```python
from build123d import *

# Parameters (mm, degrees)
SKETCH1_W           = 40
SKETCH1_H           = 40
BOSS_EXTRUDE1_DEPTH = 30
SKETCH2_R           = 19
CUT_EXTRUDE1_DEPTH  = 30
CUT_EXTRUDE1_TAPER  = 6
SKETCH3_R           = 1.5
CUT_EXTRUDE2_DEPTH  = 15
SKETCH4_W           = 24
SKETCH4_H           = 15
CUT_EXTRUDE3_DEPTH  = 41
SKETCH5_W           = 30
SKETCH5_H           = 25
CUT_EXTRUDE4_DEPTH  = 15
SKETCH7_R           = 1.75
BOSS_EXTRUDE2_DEPTH = 5
FILLET1_R           = 10
FILLET2_R           = 10


with BuildPart() as part:
    # Sketch1 → Boss-Extrude1 (new body)
    with BuildSketch(Plane(origin=(0, 0, 0), x_dir=(1, 0, 0), z_dir=(0, 1, 0))):
        Rectangle(SKETCH1_W, SKETCH1_H)
    extrude(amount=BOSS_EXTRUDE1_DEPTH)

    # Sketch2 → Cut-Extrude1 (cut)
    with BuildSketch(Plane(origin=(0, 30, 0), x_dir=(1, 0, 0), z_dir=(0, 1, 0))):
        Circle(SKETCH2_R)
    extrude(amount=-CUT_EXTRUDE1_DEPTH, taper=CUT_EXTRUDE1_TAPER, mode=Mode.SUBTRACT)

    # Sketch3 → Cut-Extrude2 (cut)
    with BuildSketch(Plane(origin=(0, 30, 0), x_dir=(1, 0, 0), z_dir=(0, 1, 0))):
        with Locations((-15.810907627, 15.810907627)):
            Circle(SKETCH3_R)
        with Locations((16.189092373, 15.810907627)):
            Circle(SKETCH3_R)
        with Locations((16.189092373, -16.189092373)):
            Circle(SKETCH3_R)
        with Locations((-15.810907627, -16.189092373)):
            Circle(SKETCH3_R)
    extrude(amount=-CUT_EXTRUDE2_DEPTH, mode=Mode.SUBTRACT)

    # Sketch4 → Cut-Extrude3 (cut, through all)
    with BuildSketch(Plane(origin=(0, 0, -20), x_dir=(-1, 0, 0), z_dir=(0, 0, -1))):
        with Locations((0, 7.5)):
            Rectangle(SKETCH4_W, SKETCH4_H)
    extrude(amount=-CUT_EXTRUDE3_DEPTH, mode=Mode.SUBTRACT)

    # Sketch5 → Cut-Extrude4 (cut)
    with BuildSketch(Plane.XY.offset(20)):
        with Locations((0, 12.5)):
            Rectangle(SKETCH5_W, SKETCH5_H)
    extrude(amount=-CUT_EXTRUDE4_DEPTH, mode=Mode.SUBTRACT)

    # Sketch7 → Boss-Extrude2 (add)
    with BuildSketch(Plane.XZ):
        with BuildLine():
            Line((-20, 3), (-20, -3))
            ThreePointArc((-20, -3), (-29, 0), (-20, 3))
        make_face()
        with Locations((-24, 0)):
            Circle(SKETCH7_R, mode=Mode.SUBTRACT)
        with BuildLine():
            Line((20, 3), (20, -3))
            ThreePointArc((20, -3), (29, 0), (20, 3))
        make_face()
        with Locations((24, 0)):
            Circle(SKETCH7_R, mode=Mode.SUBTRACT)
    extrude(amount=-BOSS_EXTRUDE2_DEPTH)

    # Fillet1
    fillet1_edges = [part.edges().sort_by_distance(p)[0] for p in [
        (-20, 2.5, 3),
    ]]
    fillet(fillet1_edges, radius=FILLET1_R)

    # Fillet2
    fillet2_edges = [part.edges().sort_by_distance(p)[0] for p in [
        (-20, 2.5, -3),
        (20, 2.5, 3),
        (20, 2.5, -3),
    ]]
    fillet(fillet2_edges, radius=FILLET2_R)


solid = part.part
```
The model under review builds one solid part; all positions refer to its coordinate system, in mm. A direction names the side the tool comes from. Round coordinates to 2 decimals unless told otherwise and drop trailing zeros. Order: outer loops, then holes, each group sorted by start corner. A loop starts at its lowest first (then second) coordinate and runs counter-clockwise, first axis right, second up. Notation, with made-up numbers: (25, -25) -> (38, -25) arc R36 cw to (38, 14) -> close; hole circle Ø10 at (55.5, -14). An arc over 180 degrees is marked (long way). One line per item, written item: value. Start each with the question number.
Q1. Take a section at A-A (y = 2.5). Write out the cut boundary in (x, z).
Q2. Wall thickness on line 1 (X direction, y = 7, z = 18); line 2 (X direction, y = 21, z = -15); line 3 (Z direction, x = 16, y = 26): over which ranges is each line inside the solid? List them lowest first.
Q3. Clearance check with flat-ended pins moving along their axes: pin 1 Ø15 at (y, z) = (21.5, -8.5) entering from +X; pin 2 Ø4 at (x, z) = (16.19, -15.81) entering from +Y; pin 3 Ø7 at (x, z) = (-25.5, 5.5) entering from +Y; pin 4 Ø12 at (y, z) = (9.5, 7) entering from +X. State where each tip first meets the part, or that it passes through.
Q4. Take a section at C-C (y = 16). Write out the cut boundary in (x, z).
Q5. Mouldability with a two-part tool opening along Z and no side actions: class faces 1 (the face through (-21.59, 2.54, -8.34)), 2 (the face through (-16, 15, 16)), 3 (the face through (-15, 10, 14)) as released by +Z, released by -Z, zero draft, split by the parting line, or undercut.
Q6. Take a section at D-D (z = 0). Count the separate pieces of the cut face and the enclosed holes in it, and give its area (3 significant figures).
Q7. Machinability: for faces 4 (the face through (15, 10, 14)), 5 (the face through (-21, 5, 0)), 6 (the face through (17.62, 22.6, 15.74)), which of the approach directions +Z, -Z, +X, -X, +Y, -Y give a long, thin tool a straight path to every point of the face, cutting with its end or side? Answer none if there is none.
Reported:
1. outline: (-26, -4.58) arc R10 cw to (-20, -13.75) -> (-20, -20) -> (-12, -20) -> (-12, -10.75) arc R16.11 cw to (-15, 5.88) -> (-15, 20) -> (-20, 20) -> (-20, 13.75) arc R10 cw to (-26, 4.58) arc R5 ccw to start; (12, -20) -> (20, -20) -> (20, -13.75) arc R10 cw to (26, -4.58) arc R5 ccw to (26, 4.58) arc R10 cw to (20, 13.75) -> (20, 20) -> (15, 20) -> (15, 5.88) arc R16.11 cw to (12, -10.75) -> close; hole circle Ø3.5 at (-24, 0); hole circle Ø3.5 at (24, 0)
2. line 1: x = -20 to -15, 15 to 20
2. line 2: x = -20 to -17.07, -14.55 to -10.05, 10.05 to 14.93, 17.45 to 20
2. line 3: z = -20 to -17.3, -14.32 to -9.44, 9.44 to 14.7, 17.68 to 20
3. pin 1: stops at x = 20
3. pin 2: stops at y = 30
3. pin 3: stops at y = 5
3. pin 4: stops at x = 27.98
4. outline: (-20, -20) -> (20, -20) -> (20, 20) -> (15, 20) -> (15, 17.1) arc R1.5 cw (long way) to (15, 15.27) -> (15, 9.07) arc R17.53 cw (long way) to (-15, 9.07) -> (-15, 14.93) arc R1.5 cw (long way) to (-15, 17.45) -> (-15, 20) -> (-20, 20) -> close; hole circle Ø3 at (-15.81, -15.81); hole circle Ø3 at (16.19, -15.81)
5. face 1: released by -Z
5. face 2: undercut
5. face 3: zero draft
6. separate pieces: 4
6. enclosed holes: 0
6. area: 210 mm2
7. face 4: +Z, -Y
7. face 5: +Z, -Z, -X, +Y
7. face 6: +Y
